Geometry: final body of the model. Coordinates: model frame, mm. A direction names the side the tool comes from. Give positions to 0.01 mm unless a question says otherwise; leave off trailing zeros. Order: outer loops, then holes, each group sorted by start corner. A loop starts at its lowest first (then second) coordinate and runs counter-clockwise, first axis right, second up. Notation, with made-up numbers: M 43,14.25 L 73,14.25 A26 ccw 73,28.25 Z; hole C 4,-23 d9. An arc over 180 degrees is marked long. Use CSV: the item, a comma, the result in double quotes.
```python
from build123d import *

# Parameters (mm, degrees)
SKETCH_R     = 3
PAD_DEPTH    = 35.2
SKETCH001_R  = 2
PAD001_DEPTH = 2
SKETCH002_R  = 3
PAD002_DEPTH = 1
SKETCH003_R  = 2
PAD003_DEPTH = 2
SKETCH004_R  = 3
PAD004_DEPTH = 1


with BuildPart() as part:
    # Sketch → Pad (new body)
    with BuildSketch(Plane.YZ):
        Circle(SKETCH_R)
    extrude(amount=PAD_DEPTH)

    # Sketch001 (on Face3 of Pad) → Pad001 (join)
    with BuildSketch(Plane.YZ.offset(35.2)):
        Circle(SKETCH001_R)
    extrude(amount=PAD001_DEPTH)

    # Sketch002 (on Face5 of Pad001) → Pad002 (join)
    with BuildSketch(Plane.YZ.offset(37.2)):
        Circle(SKETCH002_R)
    extrude(amount=PAD002_DEPTH)

    # Sketch003 (on Face7 of Pad002) → Pad003 (join)
    with BuildSketch(Plane(origin=(0, 0, 0), x_dir=(0, 1, 0), z_dir=(-1, 0, 0))):
        Circle(SKETCH003_R)
    extrude(amount=PAD003_DEPTH)

    # Sketch004 (on Face9 of Pad003) → Pad004 (join)
    with BuildSketch(Plane(origin=(-2, 0, 0), x_dir=(0, 1, 0), z_dir=(-1, 0, 0))):
        Circle(SKETCH004_R)
    extrude(amount=PAD004_DEPTH)


solid = part.part
```
1. Line query: line 1 (X direction, y = -0.6, z = 2.35); line 2 (Y direction, x = 32.5, z = 0.2); line 3 (Y direction, x = 33.5, z = -2.15). Output: solid intervals per line, ascending.
Answer:
line 1,"-3 to -2, 0 to 35.2, 37.2 to 38.2"
line 2,"-2.99 to 2.99"
line 3,"-2.09 to 2.09"
2. Section A-A, the plane y = 0. Return the cut outline in (x, z).
Answer:
outline,"M -3,-3 L -2,-3 L -2,-2 L 0,-2 L 0,-3 L 35.2,-3 L 35.2,-2 L 37.2,-2 L 37.2,-3 L 38.2,-3 L 38.2,3 L 37.2,3 L 37.2,2 L 35.2,2 L 35.2,3 L 0,3 L 0,2 L -2,2 L -2,3 L -3,3 Z"
3. Section C-C, the plane x = 12. Return the cut outline in (y, z).
Answer:
outline,"C 0,0 d6"
4. Reachability of faces 1 (the face through (37.2, 1, -2)), 2 (the face through (38.2, 0, 0)) from +Z, -Z, +X, -X, +Y, -Y: full face, straight path, thin tool, end or side. Return the list, or none.
Answer:
face 1,"none"
face 2,"+Z, -Z, +X, +Y, -Y"
